Input: part model. Units: mm. Frame: model coordinates. Face numbers are marked on the shaded views. A direction names the side the tool comes from. Give positions to 0.01 mm unless a question says otherwise; leave off trailing zeros. Order: outer loops, then holes, each group sorted by start corner. A loop starts at its lowest first (then second) coordinate and runs counter-clockwise, first axis right, second up. Notation, with made-up numbers: (5, 11.5) - (54, 11.5) arc R24 cw to (54, 21.5) - close; hole circle Ø2 at (15, 50.25). An arc over 180 degrees is marked (long way). Use a Markdown table: item, result.
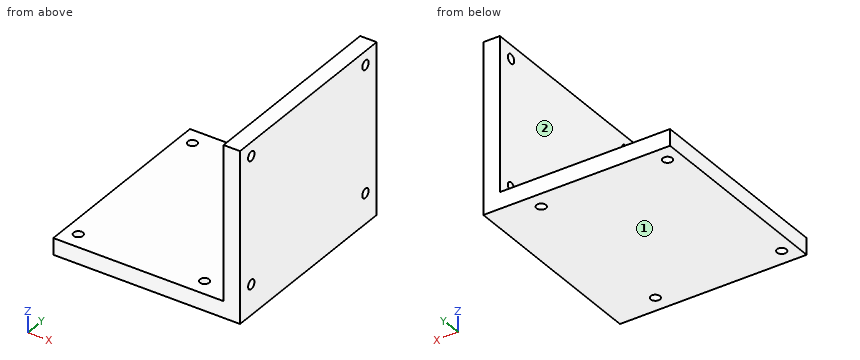
Solid Edge part; units mm, degrees
sketch "Sketch1" plane through (0, 0, 0) normal (0, 0, 1) x (1, 0, 0)
  line L0 (-28, -49) -> (40, -49)
  line L1 (40, -49) -> (40, 24)
  line L2 (40, 24) -> (-28, 24)
  line L3 (-28, 24) -> (-28, -49)
  circle A0 centre (-23, -43) radius 1.7
  circle A1 centre (23, -43) radius 1.7
  circle A2 centre (-23, 18) radius 1.7
  circle A3 centre (23, 18) radius 1.7
extrude "Protrusion1" add sketch "Sketch1" along normal blind 6
sketch "Sketch2" plane through (0, 0, 6) normal (0, 0, 1) x (1, 0, 0)
  line L0 (34, -49) -> (40, -49)
  line L1 (40, -49) -> (40, 24)
  line L2 (40, 24) -> (34, 24)
  line L3 (34, 24) -> (34, -49)
extrude "ExtrudedProtrusion_2" add sketch "Sketch2" along normal blind 56
sketch "Sketch3" plane through (34, 0, 0) normal (1, 0, 0) x (0, 1, 0)
  circle A0 centre (-43, 57) radius 1.7
  circle A1 centre (-43, 11) radius 1.7
  circle A2 centre (18, 57) radius 1.7
  circle A3 centre (18, 11) radius 1.7
extrude "ExtrudedCutout_1" cut sketch "Sketch3" along normal blind 6
1. Pin query (flat end, axial travel): pin 1 (5.5 mm diameter, centred on y = -43, z = 57, fed in from +X); pin 2 (4 mm diameter, centred on y = 18, z = 11, fed in from -X); pin 3 (3 mm diameter, centred on y = -43, z = 11, fed in from -X); pin 4 (4 mm diameter, centred on x = -3.5, y = -15, fed in from +Z). Return the tip coordinate at first contact, or that it passes through.
Response:
| item | result |
|---|---|
| pin 1 | stops at x = 40 |
| pin 2 | stops at x = 34 |
| pin 3 | passes through |
| pin 4 | stops at z = 6 |
2. Section query B-B (z = 57). Return loops of the section in (x, y).
Response:
| item | result |
|---|---|
| outline | (34, -49) - (40, -49) - (40, -44.7) - (34, -44.7) - close; (34, -41.3) - (40, -41.3) - (40, 16.3) - (34, 16.3) - close; (34, 19.7) - (40, 19.7) - (40, 24) - (34, 24) - close |
3. Section query A-A (x = -23). Return loops of the section in (y, z), then the cut area to 3 significant figures.
Response:
| item | result |
|---|---|
| outline | (-49, 0) - (-44.7, 0) - (-44.7, 6) - (-49, 6) - close; (-41.3, 0) - (16.3, 0) - (16.3, 6) - (-41.3, 6) - close; (19.7, 0) - (24, 0) - (24, 6) - (19.7, 6) - close |
| area | 397 mm^2 |
4. Material intervals for line 1 along Z through (x, y) = (36, -43); line 2 along Y through (x, z) = (-23, 1); line 3 along X through (y, z) = (16, 45), sorted ascending.
Response:
| item | result |
|---|---|
| line 1 | z = 0 to 9.3, 12.7 to 55.3, 58.7 to 62 |
| line 2 | y = -49 to -44.7, -41.3 to 16.3, 19.7 to 24 |
| line 3 | x = 34 to 40 |
5. Set-up query: the marked faces 1 and 2. Return all of +Z, -Z, +X, -X, +Y, -Y with unobstructed straight access to the full face (end or side cutting, diameter ignored); none if empty.
Response:
| item | result |
|---|---|
| face 1 | -Z, +X, -X, +Y, -Y |
| face 2 | +Z, -X, +Y, -Y |
6. Section query D-D (y = -29.5). Return loops of the section in (x, z).
Response:
| item | result |
|---|---|
| outline | (-28, 0) - (40, 0) - (40, 62) - (34, 62) - (34, 6) - (-28, 6) - close |
7. Section query C-C (y = 18). Return loops of the section in (x, z), then the cut area to 3 significant figures.
Response:
| item | result |
|---|---|
| outline | (-28, 0) - (-24.7, 0) - (-24.7, 6) - (-28, 6) - close; (-21.3, 0) - (21.3, 0) - (21.3, 6) - (-21.3, 6) - close; (24.7, 0) - (40, 0) - (40, 9.3) - (34, 9.3) - (34, 6) - (24.7, 6) - close; (34, 12.7) - (40, 12.7) - (40, 55.3) - (34, 55.3) - close; (34, 58.7) - (40, 58.7) - (40, 62) - (34, 62) - close |
| area | 662 mm^2 |
